Input: dimensioned drawing with shaded views. Units: mm. Origin: part minimum x, y, z. Round coordinates to 2 decimals unless told otherwise and drop trailing zeros. Write each loop counter-clockwise with the first axis right and the second up, starting at its lowest first coordinate (ties: lowest second). Pieces come first, ordered by that corner, then holes. Notation, with made-up numbers: (-22.5, 32) -> (1.5, 32) arc R22 cw to (1.5, 49) -> close; hole circle Ø11 at (-38, -29.5). An arc over 180 degrees is marked (long way). Use one line per item in the form item = value. Start each with the question number.
1. Cut plane C-C, the plane z = 92. State how many separate pieces and enclosed holes the cut face has, plus the area to 3 significant figures.
2. Cut plane D-D, the plane x = 156. Return the cut outline in (y, z), plus the area to 3 significant figures.
3. Pin query (flat end, axial travel): pin 1 Ø1.5 at (y, z) = (55, 143.5) entering from -X; pin 2 Ø5 at (x, z) = (115.5, 150) entering from -Y (1 decimal); pin 3 Ø10 at (y, z) = (45.5, 123) entering from -X; pin 4 Ø12 at (x, y) = (35.5, 222.5) entering from +Z. Return the tip coordinate at first contact, or that it passes through.
4. Cut plane B-B, the plane x = 105. Return the cut outline in (y, z), plus the area to 3 significant figures.
5. Draft query along X for the marked faces 1, 2, 3 and 4. Return one class per face: pulls with the +X half, pulls with the -X half, needs draft (parallel to the pull), parting line crosses it, or undercut.
6. Cut plane A-A, the plane y = 105. Return the cut outline in (x, z).
7. Line query: L1, parallel to Y at x = 105, z = 77; L2, parallel to X at y = 119, z = 46.5; L3, parallel to X at y = 90.5, z = 45 (1 decimal). Output: solid intervals per line, ascending.
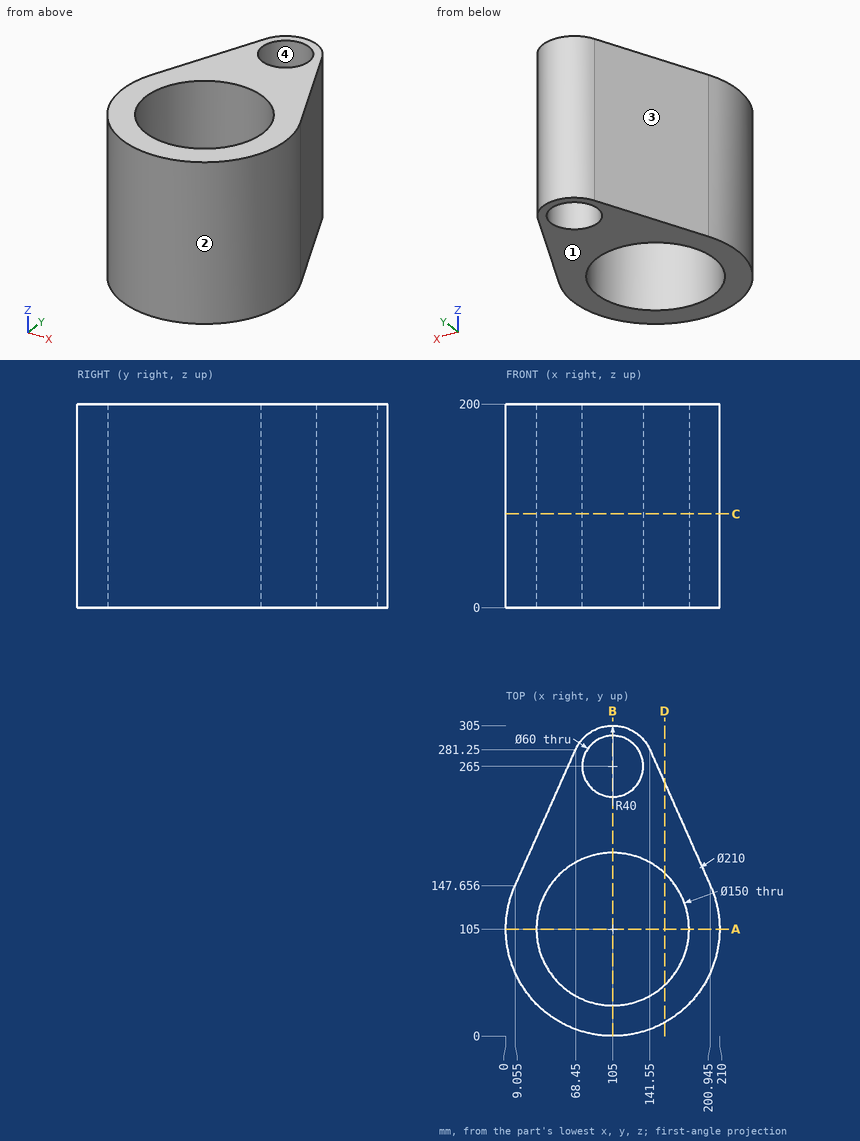
Outcome:
q1.separate_pieces = 1
q1.enclosed_holes = 2
q1.area = 24,500 mm^2
q2.outline = (13.22, 0) -> (50.01, 0) -> (50.01, 200) -> (13.22, 200) -> close; (159.99, 0) -> (248.75, 0) -> (248.75, 200) -> (159.99, 200) -> close
q2.area = 25,100 mm^2
q3.pin_1 = 12.27
q3.pin_2 = 0.3
q3.pin_3 = 15.25
q3.pin_4 = through
q4.outline = (0, 0) -> (30, 0) -> (30, 200) -> (0, 200) -> close; (180, 0) -> (235, 0) -> (235, 200) -> (180, 200) -> close; (295, 0) -> (305, 0) -> (305, 200) -> (295, 200) -> close
q4.area = 19,000 mm^2
q5.face_1 = needs draft
q5.face_2 = parting line crosses it
q5.face_3 = pulls with the -X half
q5.face_4 = undercut
q6.outline = (0, 0) -> (30, 0) -> (30, 200) -> (0, 200) -> close; (180, 0) -> (210, 0) -> (210, 200) -> (180, 200) -> close
q7.L1 = 0 to 30, 180 to 235, 295 to 305
q7.L2 = 0.94 to 31.32, 178.68 to 209.06
q7.L3 = 1 to 31.4, 178.6 to 209
